from build123d import *

# Parameters (mm, degrees)
SZKIC1_W                     = 90.5
SZKIC1_H                     = 26
DODANIE_WYCI_GNI_CIE1_DEPTH  = 0.7
DODANIE_WYCI_GNI_CIE2_DEPTH  = 90.5
DODANIE_WYCI_GNI_CIE3_DEPTH  = 0.7
DODANIE_WYCI_GNI_CIE4_DEPTH  = 0.7
SZKIC9_W                     = 1.35
SZKIC9_H                     = 26.839634362
DODANIE_WYCI_GNI_CIE5_DEPTH  = 7.9
DODANIE_WYCI_GNI_CIE6_DEPTH  = 17.3
DODANIE_WYCI_GNI_CIE7_DEPTH  = 17.3
WYTNIJ_WYCI_GNI_CIE1_START   = -0.7
WYTNIJ_WYCI_GNI_CIE1_DEPTH   = 0.7
SZKIC14_W                    = 0.7
SZKIC14_H                    = 3
DODANIE_WYCI_GNI_CIE8_DEPTH  = 3.15
DODANIE_WYCI_GNI_CIE9_DEPTH  = 0.7
SZKIC18_R                    = 2.175
WYTNIJ_WYCI_GNI_CIE2_DEPTH   = 0.7
SZKIC19_W                    = 8.5
SZKIC19_H                    = 2
DODANIE_WYCI_GNI_CIE10_DEPTH = 0.7
WYTNIJ_WYCI_GNI_CIE3_DEPTH   = 0.7
SZKIC22_W                    = 3.6
SZKIC22_H                    = 0.7
DODANIE_WYCI_GNI_CIE11_DEPTH = 3.3
SZKIC23_R                    = 2.5
WYTNIJ_WYCI_GNI_CIE4_DEPTH   = 0.7


with BuildPart() as part:
    # Szkic1 → Dodanie-wyci_gni_cie1 (new body)
    with BuildSketch(Plane.XY):
        with Locations((8.895925444, -12.413393351)):
            Rectangle(SZKIC1_W, SZKIC1_H)
    extrude(amount=DODANIE_WYCI_GNI_CIE1_DEPTH)



with BuildPart() as body_2:
    # Szkic3 → Dodanie-wyci_gni_cie2 (new body)
    with BuildSketch(Plane.ZY.offset(36.354074556)):
        with BuildLine():
            Line((5.5, -26.413393351), (5.5, -26.670245495))
            ThreePointArc((5.5, -26.670245495), (5.249678176, -27.332048058), (4.624034735, -27.662523372))
            Line((4.624034735, -27.662523372), (-6.01042337, -28.991830635))
            Line((-6.01042337, -28.991830635), (-6.097247684, -28.297236121))
            Line((-6.097247684, -28.297236121), (4.497633639, -26.977852669))
            ThreePointArc((4.497633639, -26.977852669), (4.713586161, -26.863878738), (4.8, -26.635497046))
            Line((4.8, -26.635497046), (4.8, -26.598027713))
            ThreePointArc((4.8, -26.598027713), (4.69895184, -26.354075874), (4.455, -26.253027713))
            Line((4.455, -26.253027713), (0, -26.253027713))
            Line((0, -26.253027713), (0, -25.413393351))
            Line((0, -25.413393351), (4.5, -25.413393351))
            ThreePointArc((4.5, -25.413393351), (5.207106781, -25.706286569), (5.5, -26.413393351))
        make_face()
    extrude(amount=-DODANIE_WYCI_GNI_CIE2_DEPTH)


with BuildPart() as part_1:
    add(part.part)

    add(body_2.part)  # Dodanie-wyci_gni_cie3 merges body 2
    # Szkic4 → Dodanie-wyci_gni_cie3 (add)
    with BuildSketch(Plane(origin=(54.145925444, 0, 0), x_dir=(0, 0, -1), z_dir=(1, 0, 0))):
        with BuildLine():
            Line((0, 0.586606649), (-4.796894469, 0.586606649))
            ThreePointArc((-4.796894469, 0.586606649), (-6.277718772, -0.069087068), (-6.787575884, -1.606233969))
            add(Edge.make_bspline(
                [(-4.469267418, -27.681869286), (-4.44254495, -27.204916247), (-4.010367743, -18.290006756), (-4.851145038, -9.610716303), (-6.787575884, -1.606233969)],
                knots=[-0.045928805, -0.045928805, -0.045928805, -0.045928805, 0, 0.813756029, 0.813756029, 0.813756029, 0.813756029], degree=3))
            Line((-4.469267418, -27.681869286), (0, -28.240527713))
            Line((0, -28.240527713), (0, 0.586606649))
        make_face()
    extrude(amount=DODANIE_WYCI_GNI_CIE3_DEPTH)

    # Szkic8 → Dodanie-wyci_gni_cie4 (add)
    with BuildSketch(Plane.ZY.offset(36.354074556)):
        with BuildLine():
            Line((4.469267418, -27.681869286), (0, -28.240527713))
            Line((0, -28.240527713), (0, 0.586606649))
            Line((0, 0.586606649), (4.796894469, 0.586606649))
            ThreePointArc((4.796894469, 0.586606649), (6.277718772, -0.069087068), (6.787575884, -1.606233969))
            add(Edge.make_bspline(
                [(4.469267418, -27.681869286), (4.44254495, -27.204916247), (4.010367743, -18.290006756), (4.851145038, -9.610716303), (6.787575884, -1.606233969)],
                knots=[-0.045928805, -0.045928805, -0.045928805, -0.045928805, 0, 0.813756029, 0.813756029, 0.813756029, 0.813756029], degree=3))
        make_face()
    extrude(amount=DODANIE_WYCI_GNI_CIE4_DEPTH)

    # Szkic9 → Dodanie-wyci_gni_cie5 (add)
    with BuildSketch(Plane(origin=(0, 0, 0), x_dir=(-1, 0, 0), z_dir=(0, 0, -1))):
        with Locations((-54.170925444, -12.833210532)):
            Rectangle(SZKIC9_W, SZKIC9_H)
        with Locations((36.379074556, -12.833210532)):
            Rectangle(SZKIC9_W, SZKIC9_H)
    extrude(amount=DODANIE_WYCI_GNI_CIE5_DEPTH)

    # Szkic11 → Dodanie-wyci_gni_cie6 (add)
    with BuildSketch(Plane(origin=(0, 0.586606649, 0), x_dir=(1, 0, 0), z_dir=(0, 1, 0))):
        Polygon((-37.054074556, 7.9), (-37.054074556, 7.2), (-44.354074556, 7.2), (-44.354074556, 17.2), (-55.654074556, 17.2), (-55.654074556, 17.9), (-43.654074556, 17.9), (-43.654074556, 7.9), align=None)
    extrude(amount=-DODANIE_WYCI_GNI_CIE6_DEPTH)

    # Szkic12 → Dodanie-wyci_gni_cie7 (add)
    with BuildSketch(Plane(origin=(0, 0.586606649, 0), x_dir=(1, 0, 0), z_dir=(0, 1, 0))):
        Polygon((54.845925444, 7.9), (54.845925444, 7.2), (62.145925444, 7.2), (62.145925444, 23.88), (74.265925444, 23.88), (74.265925444, 24.58), (61.445925444, 24.58), (61.445925444, 7.9), align=None)
    extrude(amount=-DODANIE_WYCI_GNI_CIE7_DEPTH)

    # Szkic13 → Wytnij-wyci_gni_cie1 (cut)
    with BuildSketch(Plane.XY.offset(-23.88).offset(WYTNIJ_WYCI_GNI_CIE1_START)):
        Polygon((67.004736449, 0.586606649), (75.489507901, -5.272079996), (69.539548838, -16.713393351), (76.249870064, -16.713393351), (76.249870064, 0.586606649), align=None)
        with BuildLine():
            Line((62.145925444, -4.163393351), (66.176231598, -4.163393351))
            ThreePointArc((66.176231598, -4.163393351), (69.745925444, -5.663393351), (66.176231598, -7.163393351))
            Line((66.176231598, -7.163393351), (62.145925444, -7.163393351))
            Line((62.145925444, -7.163393351), (62.145925444, -4.163393351))
        make_face()
    extrude(amount=WYTNIJ_WYCI_GNI_CIE1_DEPTH, mode=Mode.SUBTRACT)

    # Szkic14 → Dodanie-wyci_gni_cie8 (add)
    with BuildSketch(Plane(origin=(0, 0, -24.58), x_dir=(-1, 0, 0), z_dir=(0, 0, -1))):
        with Locations((-61.795925444, -5.663393351)):
            Rectangle(SZKIC14_W, SZKIC14_H)
    extrude(amount=DODANIE_WYCI_GNI_CIE8_DEPTH)

    # Szkic17 → Dodanie-wyci_gni_cie9 (add)
    with BuildSketch(Plane.XY.offset(-17.2)):
        Polygon((-44.353275943, 0.54213061), (-55.654074556, 0.586606649), (-55.654074556, 5.586606649), (-44.353275943, 5.586606649), align=None)
    extrude(amount=-DODANIE_WYCI_GNI_CIE9_DEPTH)

    # Szkic18 → Wytnij-wyci_gni_cie2 (cut)
    with BuildSketch(Plane.XY.offset(-17.2)):
        with Locations((-49.249074556, -0.088393351)):
            Circle(SZKIC18_R)
        Polygon((-51.424074556, 5.586606649), (-55.654074556, 2.286606649), (-55.654074556, 5.586606649), align=None)
        with BuildLine():
            Line((-55.654074556, -4.413393351), (-52.654074556, -4.413393351))
            ThreePointArc((-52.654074556, -4.413393351), (-50.886307603, -5.145626398), (-50.154074556, -6.913393351))
            Line((-50.154074556, -6.913393351), (-50.154074556, -7.413393351))
            ThreePointArc((-50.154074556, -7.413393351), (-50.886307603, -9.181160304), (-52.654074556, -9.913393351))
            Line((-52.654074556, -9.913393351), (-55.654074556, -9.913393351))
            Line((-55.654074556, -9.913393351), (-55.654074556, -4.413393351))
        make_face()
    extrude(amount=-WYTNIJ_WYCI_GNI_CIE2_DEPTH, mode=Mode.SUBTRACT)

    # Szkic19 → Dodanie-wyci_gni_cie10 (add)
    with BuildSketch(Plane.XY.offset(-17.2)):
        with Locations((-51.404074556, -17.713393351)):
            Rectangle(SZKIC19_W, SZKIC19_H)
    extrude(amount=-DODANIE_WYCI_GNI_CIE10_DEPTH)

    # Szkic21 → Wytnij-wyci_gni_cie3 (cut)
    with BuildSketch(Plane.XY.offset(-17.2)):
        Polygon((-55.654074556, -13.813393351), (-50.754074556, -18.713393351), (-55.654074556, -18.713393351), align=None)
    extrude(amount=-WYTNIJ_WYCI_GNI_CIE3_DEPTH, mode=Mode.SUBTRACT)

    # Szkic22 → Dodanie-wyci_gni_cie11 (add)
    with BuildSketch(Plane(origin=(0, 0, -17.9), x_dir=(-1, 0, 0), z_dir=(0, 0, -1))):
        with Locations((48.954074556, -18.363393351)):
            Rectangle(SZKIC22_W, SZKIC22_H)
    extrude(amount=DODANIE_WYCI_GNI_CIE11_DEPTH)

    # Szkic23 → Wytnij-wyci_gni_cie4 (cut)
    with BuildSketch(Plane(origin=(0, 0, 0), x_dir=(-1, 0, 0), z_dir=(0, 0, -1))):
        with Locations((-48.950925444, -5.101869726)):
            Circle(SZKIC23_R)
        with Locations((30.424074556, -5.101869726)):
            Circle(SZKIC23_R)
        with Locations((-48.950925444, -18.436869726)):
            Circle(SZKIC23_R)
    extrude(amount=-WYTNIJ_WYCI_GNI_CIE4_DEPTH, mode=Mode.SUBTRACT)


solid = part_1.part
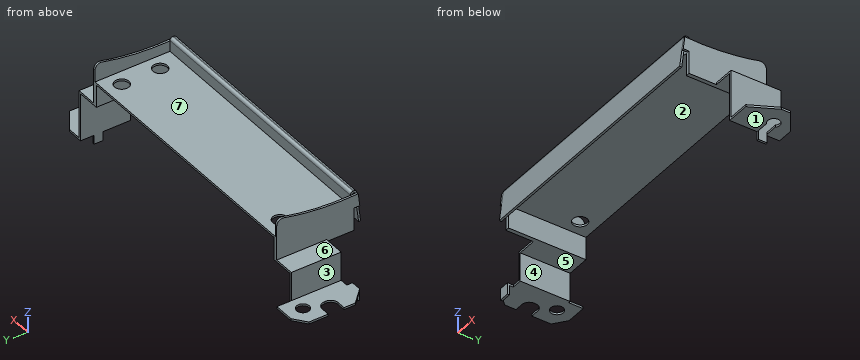
Source: CAD feature listing. Evaluate the final solid. Frame: model axes, mm. Face numbers are marked on the shaded views. A direction names the side the tool comes from. Round coordinates to 2 decimals unless told otherwise and drop trailing zeros. Loops run counter-clockwise (first coordinate to the right, second up) from the corner with the lowest first, then second, coordinate; pieces in that order, holes last. Notation, with made-up numbers: (-5, 80.25) -> (9, 80.25) arc R30 ccw to (9, 116.25) -> close; hole circle Ø2 at (-10.75, 8.25). An arc over 180 degrees is marked (long way). Answer as a JSON object with one key per item and string values. Group by question number.
Q1. Contact query for flat-ended pins moving along their axis: P1, Ø8, axis at x = 24.5, y = -1.5, coming from the +Z side; P2, Ø1, axis at y = 1.5, z = -17, coming from the -X side; P3, Ø1, axis at y = -10, z = -20.5, coming from the +X side; P4, Ø1, axis at x = 13.5, y = -10.5, coming from the -Z side. Output: stop coordinate, or through.
Q2. Section query A-A (z = -10). Output: boundary loops of the cut face in (x, y).
Q3. Ray query, line 1 (X direction, y = -13.5, z = 1); line 2 (X direction, y = -10.5, z = -6); line 3 (Z direction, x = 7, y = -3). Return the intervals inside material, ascending. Write a range as from..to.
Q4. Mould query, pull axis X, two halves, no side actions, for the marked faces 1, 2, 3 and 4. Classes: pulls with the +X half, pulls with the -X half, needs draft (parallel to the pull), parting line crosses it, or undercut.
Q5. Section query C-C (z = -4). Output: boundary loops of the cut face in (x, y), plus the area to 3 significant figures.
Q6. Access query for the marked faces 5, 6 and 7. Directions: +Z, -Z, +X, -X, +Y, -Y. A direction counts if a zero-diameter tool reaches every point of the face in a straight line with its end or side. Return the directions, or none.
Completed:
{
 "1": {"P1": "z = 0.7", "P2": "x = -55.65", "P3": "x = 62.15", "P4": "z = 0"},
 "2": {"outline": "(-44.35, -16.71) -> (-43.65, -16.71) -> (-43.65, 0.59) -> (-44.35, 0.59) -> close; (61.45, -16.71) -> (62.15, -16.71) -> (62.15, 0.59) -> (61.45, 0.59) -> close"},
 "3": {"line 1": "-37.05..-36.35, 54.15..54.85", "line 2": "-37.05..-35.7, 53.5..54.85", "line 3": "0..0.7"},
 "4": {"face 1": "needs draft", "face 2": "undercut", "face 3": "pulls with the -X half", "face 4": "undercut"},
 "5": {"outline": "(-37.05, -26.25) -> (-35.7, -26.25) -> (-35.7, 0.59) -> (-37.05, 0.59) -> close; (-36.35, -28.74) -> (54.15, -28.74) -> (54.15, -28.04) -> (-36.35, -28.04) -> close; (53.5, -26.25) -> (54.85, -26.25) -> (54.85, 0.59) -> (53.5, 0.59) -> close", "area": "136 mm²"},
 "6": {"face 5": "-Z, +Y, -Y", "face 6": "+Z, -X, +Y, -Y", "face 7": "+Z, +Y"}
}
